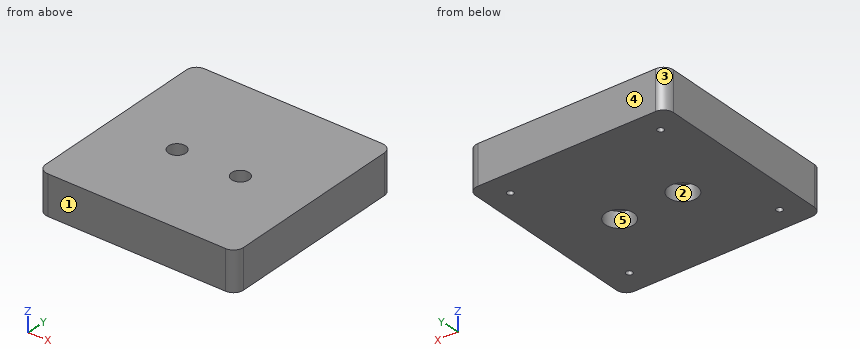
from build123d import *

# Parameters (mm, degrees)
F1_DEPTH       = 20
F3_D           = 8.8
F3_CBORE_D     = 14.25
F3_CBORE_DEPTH = 8
F5_D           = 3.2
F5_DEPTH       = 15
F5_TIP         = 0.9613769904


with BuildPart() as f1:
    # F0 (on Top) → F1 (new body)
    with BuildSketch(Plane.XY):
        with BuildLine():
            ThreePointArc((-50, -45), (-48.5355339059, -48.5355339059), (-45, -50))
            Line((-45, -50), (45, -50))
            ThreePointArc((45, -50), (48.5355339059, -48.5355339059), (50, -45))
            Line((50, -45), (50, 45))
            ThreePointArc((50, 45), (48.5355339059, 48.5355339059), (45, 50))
            Line((45, 50), (-45, 50))
            ThreePointArc((-45, 50), (-48.5355339059, 48.5355339059), (-50, 45))
            Line((-50, 45), (-50, -45))
        make_face()
    extrude(amount=F1_DEPTH)

    # F3 (through all)
    with Locations(Plane(origin=(0, 0, 0), x_dir=(1, 0, 0), z_dir=(0, 0, -1))):
        with Locations((-16, 4), (16, 4)):
            CounterBoreHole(F3_D / 2, F3_CBORE_D / 2, F3_CBORE_DEPTH)

    # F5
    with Locations(Plane(origin=(0, 0, 0), x_dir=(1, 0, 0), z_dir=(0, 0, -1))):
        with Locations((-38, 38), (38, 38), (38, -38), (-38, -38)):
            Hole(F5_D / 2, depth=F5_DEPTH)
            with Locations((0, 0, -(F5_DEPTH + F5_TIP / 2))):  # 118° drill point
                Cone(0, F5_D / 2, F5_TIP, mode=Mode.SUBTRACT)


solid = f1.part
The model under review builds one solid part; all positions refer to its coordinate system, in mm. Face numbers are marked on the shaded views. A direction names the side the tool comes from. Round coordinates to 2 decimals unless told otherwise and drop trailing zeros. Order: outer loops, then holes, each group sorted by start corner. A loop starts at its lowest first (then second) coordinate and runs counter-clockwise, first axis right, second up. Notation, with made-up numbers: (-36, 59) -> (-19, 59) arc R28 cw to (-19, 86) -> close; hole circle Ø7 at (-40, -29.5). An arc over 180 degrees is marked (long way). Use CSV: the item, a comma, the result in double quotes. Start each with the question number.
(1) Wall thickness on probe 1 along Y at (x, z) = (-38, 7); probe 2 along Y at (x, z) = (-16, 2.5) (3 decimals): over which ranges is each line inside the solid? List them lowest first. Write a range as from..to.
(2) Consider section C-C on x = 13.5. Write out the cut boundary in (y, z), and give its area (3 significant figures).
(3) Tool access review of the marked faces 1 and 2: name each direction out of +Z, -Z, +X, -X, +Y, -Y from which nothing blocks a thin tool from reaching the whole face with its end or side.
(4) Consider section B-B on x = -16. Write out the cut boundary in (y, z) (3 decimals).
(5) Consider section A-A on z = 13.5. Write out the cut boundary in (x, y).
(6) Insertion check: pin 1 (4.5 mm diameter, centred on x = 14.5, y = -2, fed in from -Z). The pin has a flat end and moves straight along its axis. Give the tip position at first contact, or say it passes through.
(7) Mouldability with a two-part tool opening along X and no side actions: class the marked faces 3, 4 and 5 as pulls with the +X half, pulls with the -X half, needs draft (parallel to the pull), parting line crosses it, or undercut.
Responses:
1,probe 1,"-50..-39.6, -36.4..36.4, 39.6..50"
1,probe 2,"-50..-11.125, 3.125..50"
2,outline,"(-50, 0) -> (-10.67, 0) -> (-10.67, 8) -> (-7.62, 8) -> (-7.62, 20) -> (-50, 20) -> close; (-0.38, 8) -> (2.67, 8) -> (2.67, 0) -> (50, 0) -> (50, 20) -> (-0.38, 20) -> close"
2,area,"1,810 mm²"
3,face 1,"+Z, -Z, +X, -X, -Y"
3,face 2,"-Z"
4,outline,"(-50, 0) -> (-11.125, 0) -> (-11.125, 8) -> (-8.4, 8) -> (-8.4, 20) -> (-50, 20) -> close; (0.4, 8) -> (3.125, 8) -> (3.125, 0) -> (50, 0) -> (50, 20) -> (0.4, 20) -> close"
5,outline,"(-50, -45) arc R5 ccw to (-45, -50) -> (45, -50) arc R5 ccw to (50, -45) -> (50, 45) arc R5 ccw to (45, 50) -> (-45, 50) arc R5 ccw to (-50, 45) -> close; hole circle Ø3.2 at (-38, -38); hole circle Ø3.2 at (-38, 38); hole circle Ø8.8 at (-16, -4); hole circle Ø8.8 at (16, -4); hole circle Ø3.2 at (38, -38); hole circle Ø3.2 at (38, 38)"
6,pin 1,"z = 8"
7,face 3,"pulls with the -X half"
7,face 4,"needs draft"
7,face 5,"undercut"
